Can you work these out from the model? Positions are in its coordinate system, mm. A direction names the side the tool comes from. Coordinates: 2 decimals unless noted, no trailing zeros. Use a Markdown table: item, result. Add a question column.
1. For faces 1 (the cylindrical face through (-40.445, 2.37, -42.65)), 2 (the cylindrical face through (-38.172, 0.783, -45.782)), which set-ups out of +Z, -Z, +X, -X, +Y, -Y let a thin tool reach every point of the face, with its end or its side?
2. For pin 1 Ø5 at (x, z) = (-6.35, -6.35) entering from +Y; pin 2 Ø1.5 at (y, z) = (2, -5.5) entering from -X; pin 3 Ø1 at (x, y) = (-36, 2) entering from +Z, each with a flat end and sliding along its axis, tell me the tip position at first contact or that it passes through.
3. We'd pull the mould along Z, two halves only. Please class faces 3 (the flat face through (-12, 0, -25)), 4 (the cylindrical face through (-7.2, 2.4, -3.7)), 5 (the cylindrical face through (-21.91, 2.22, -49.59)), 6 (the flat face through (-5, 1.588, -5)): pulls with the +Z half, pulls with the -Z half, needs draft (parallel to the pull), parting line crosses it, or undercut.
4. Suppose I cut it at C-C, the plane y = 2.1. State how many separate pieces and enclosed holes the cut face has, then the cut area to 3 significant figures.
5. If I drill on line 1 along Z through (x, y) = (-23, 2.3); line 2 along X through (y, z) = (0.5, -19); line 3 along X through (y, z) = (2.3, -43), over which ranges is the centre line in solid material (lowest first)? Write a range as from..to.
Autodesk Inventor part; units mm, degrees
ref_plane "YZ Plane" through (0, 0, 0) normal (1, 0, 0) x (0, 1, 0)
ref_plane "XZ Plane" through (0, 0, 0) normal (0, 1, 0) x (-1, 0, 0)
ref_plane "XY Plane" through (0, 0, 0) normal (0, 0, 1) x (1, 0, 0)
sketch "Sketch1" plane through (0, 0, 0) normal (0, 1, 0) x (-1, 0, 0)
  line L0 (0, 0) -> (44.45, 0)
  line L1 (44.45, 0) -> (44.45, -50.4952)
  line L2 (44.45, -50.4952) -> (0, -50.4952)
  line L3 (0, -50.4952) -> (0, 0)
  dimension "d0" = 44.45
  dimension "d1" = 50.4952
extrude "Extrusion1" add sketch "Sketch1" along normal blind 3.175
sketch "Sketch2" plane through (0, 3.175, 0) normal (0, 1, 0) x (1, 0, 0)
  line L0 (-44.45, 50.4952) -> (-44.45, 0)
  line L1 (-44.45, 50.4952) -> (-38.1, 50.4952)
  line L2 (0, 50.4952) -> (-44.45, 50.4952)
  line L3 (-38.1, 50.4952) -> (-38.1, 44.1452)
  line L4 (-44.45, 0) -> (0, 0)
  line L5 (0, 0) -> (-6.35, 0)
  line L6 (-6.35, 0) -> (-6.35, 6.35)
  line L7 (-44.45, 50.4952) -> (-44.45, 25.2476)
  line L8 (-44.45, 25.2476) -> (-25.4, 25.2476)
  circle A0 centre (-25.4, 25.2476) radius 11.1125
  dimension "d4" = 6.35
  dimension "d5" = 6.35
  dimension "d6" = 6.35
  dimension "d7" = 6.35
  dimension "d15" = 25.2476
  dimension "d16" = 19.05
  dimension "d17" = 22.225
hole "Hole1" at (-6.35, 3.175, -6.35) at (-38.1, 3.175, -44.1452) direction (0, -1, 0) diameter 3.2766 depth 12.7 tip angle 118 counterbore diameter 5.5626 counterbore depth 1.5875
extrude "Extrusion2" cut sketch "Sketch2" against normal blind 3.175
fillet "Fillet1" radius 3.175 4 edges at (-44.45, 3.175, -25.2476) (-22.225, 3.175, -50.4952) (0, 3.175, -25.2476) (-22.225, 3.175, 0)
properties part number "sample holder lid for neutron r1"
Worked out:
| question | item | result |
|---|---|---|
| 1 | face 1 | +Y |
| 1 | face 2 | +Y, -Y |
| 2 | pin 1 | stops at y = 1.59 |
| 2 | pin 2 | stops at x = -44.19 |
| 2 | pin 3 | stops at z = -0.38 |
| 3 | face 3 | needs draft |
| 3 | face 4 | undercut |
| 3 | face 5 | pulls with the -Z half |
| 3 | face 6 | undercut |
| 4 | separate pieces | 1 |
| 4 | enclosed holes | 3 |
| 4 | area | 1,660 mm² |
| 5 | line 1 | z = -49.51..-36.1, -14.4..-0.99 |
| 5 | line 2 | x = -44.41..-34.59, -16.21..-0.04 |
| 5 | line 3 | x = -43.46..-40.63, -35.57..-0.99 |
